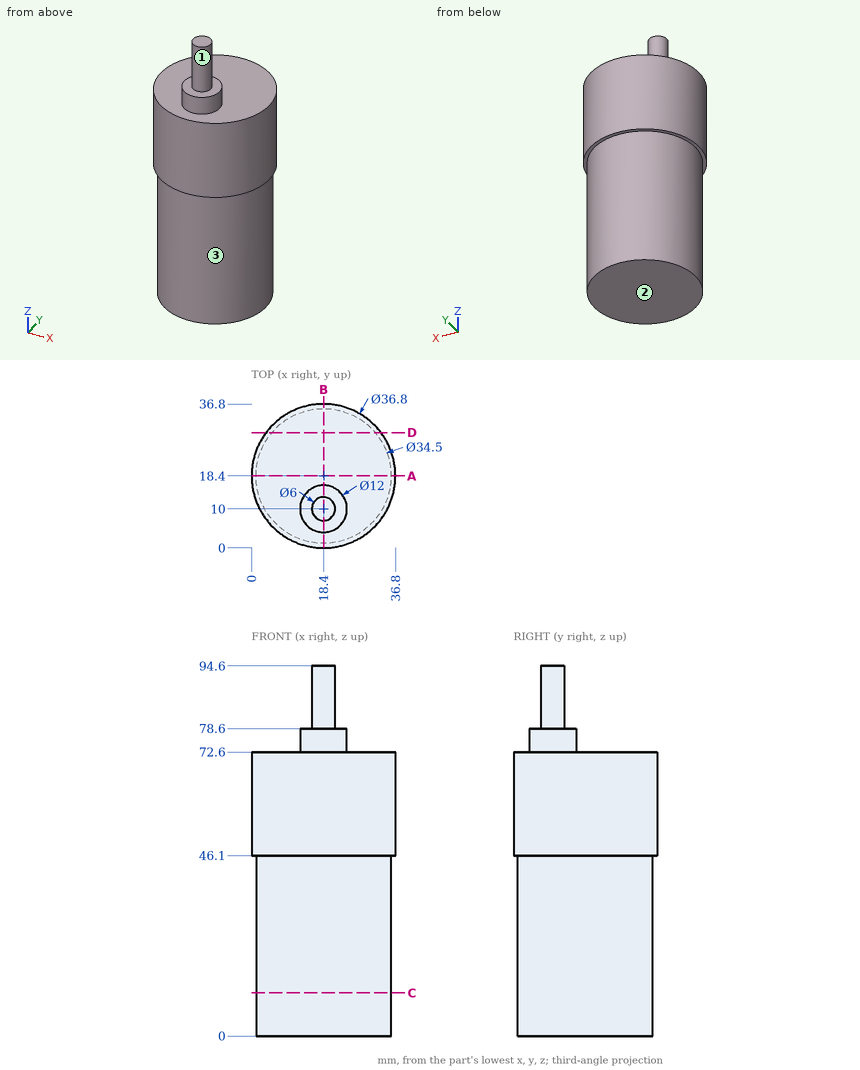
Geometry: see drawing. Coordinates: mm, zero at the bounding-box minimum. A direction names the side the tool comes from. Coordinates: 2 decimals unless noted, no trailing zeros. Loops run counter-clockwise (first coordinate to the right, second up) from the corner with the lowest first, then second, coordinate; pieces in that order, holes last. Notation, with made-up numbers: M 23.5,8 L 47.5,8 A21 cw 47.5,39 Z; hole C 55.25,61 d4. An arc over 180 degrees is marked long. Answer in a Markdown table with one row per item.
Q1. Section A-A on y = 18.4. Return the cut outline in (x, z), plus the area to 3 significant figures.
Answers below:
| item | result |
|---|---|
| outline | M 0,46.1 L 1.15,46.1 L 1.15,0 L 35.65,0 L 35.65,46.1 L 36.8,46.1 L 36.8,72.6 L 0,72.6 Z |
| area | 2,570 mm^2 |
Q2. First-contact query: pin 1 (10 mm diameter, centred on x = 7, z = 48, fed in from +Y); pin 2 (1.5 mm diameter, centred on y = 11, z = 20, fed in from +X); pin 3 (8 mm diameter, centred on y = 10.5, z = 37.5, fed in from -X); pin 4 (1.5 mm diameter, centred on y = 4.5, z = 82, fed in from +X). Flat tips, straight axial feed; report the tip coordinate or a pass-through.
Answers below:
| item | result |
|---|---|
| pin 1 | stops at y = 35.65 |
| pin 2 | stops at x = 34.32 |
| pin 3 | stops at x = 1.6 |
| pin 4 | passes through |
Q3. Section C-C on z = 11. Return the cut outline in (x, y), plus the area to 3 significant figures.
Answers below:
| item | result |
|---|---|
| outline | C 18.4,18.4 d34.5 |
| area | 935 mm^2 |
Q4. Section D-D on y = 29.5. Return the cut outline in (x, z), plus the area to 3 significant figures.
Answers below:
| item | result |
|---|---|
| outline | M 3.73,46.1 L 5.2,46.1 L 5.2,0 L 31.6,0 L 31.6,46.1 L 33.07,46.1 L 33.07,72.6 L 3.73,72.6 Z |
| area | 2,000 mm^2 |
Q5. Section B-B on x = 18.4. Return the cut outline in (y, z), plus the area to 3 significant figures.
Answers below:
| item | result |
|---|---|
| outline | M 0,46.1 L 1.15,46.1 L 1.15,0 L 35.65,0 L 35.65,46.1 L 36.8,46.1 L 36.8,72.6 L 16,72.6 L 16,78.6 L 13,78.6 L 13,94.6 L 7,94.6 L 7,78.6 L 4,78.6 L 4,72.6 L 0,72.6 Z |
| area | 2,730 mm^2 |
Q6. Set-up query: the marked faces 1, 2 and 3. Return all of +Z, -Z, +X, -X, +Y, -Y with unobstructed straight access to the full face (end or side cutting, diameter ignored); none if empty.
Answers below:
| item | result |
|---|---|
| face 1 | +Z |
| face 2 | -Z, +X, -X, +Y, -Y |
| face 3 | -Z |
Q7. Ray query, probe 1 along Z at (x, y) = (14, 7); probe 2 along Z at (x, y) = (5.5, 7); probe 3 along Y at (x, z) = (21.5, 72). Return the intervals inside material, ascending. Write a range as from..to.
Answers below:
| item | result |
|---|---|
| probe 1 | z = 0..78.6 |
| probe 2 | z = 0..72.6 |
| probe 3 | y = 0.26..36.54 |
